```python
from build123d import *

# Parameters (mm, degrees)
SCHIZZO1_W                   = 100
SCHIZZO1_H                   = 50
ESTRUSIONE_ESTRUSIONE1_DEPTH = 2
RACCORDO1_R                  = 1
RACCORDO2_R                  = 1
SCHIZZO2_W                   = 15
SCHIZZO2_H                   = 9
TAGLIO_ESTRUSIONE1_DEPTH     = 10


with BuildPart() as part:
    # Schizzo1 → Estrusione-Estrusione1 (new body)
    with BuildSketch(Plane(origin=(0, 0, 0), x_dir=(1, 0, 0), z_dir=(0, 1, 0))):
        Rectangle(SCHIZZO1_W, SCHIZZO1_H)
    extrude(amount=ESTRUSIONE_ESTRUSIONE1_DEPTH)

    # Raccordo1
    raccordo1_edges = [part.edges().sort_by_distance(p)[0] for p in [
        (0, 0, -25),
        (0, 2, -25),
    ]]
    fillet(raccordo1_edges, radius=RACCORDO1_R - 0.0001)  # a hair under: the kernel refuses the full size

    # Raccordo2
    raccordo2_edges = [part.edges().sort_by_distance(p)[0] for p in [
        (50, 0.292863929, -24.707136071),
        (50, 1.707136071, -24.707136071),
        (50, 0, 0.49995),
        (50, 2, 0.49995),
    ]]
    fillet(raccordo2_edges, radius=RACCORDO2_R - 0.0001)  # a hair under: the kernel refuses the full size

    # Schizzo2 → Taglio-Estrusione1 (cut)
    with BuildSketch(Plane(origin=(0, 2, 0), x_dir=(1, 0, 0), z_dir=(0, 1, 0))):
        with Locations((-0.220921897, -5.005960214)):
            Rectangle(SCHIZZO2_W, SCHIZZO2_H)
    extrude(amount=-TAGLIO_ESTRUSIONE1_DEPTH, mode=Mode.SUBTRACT)


solid = part.part
```
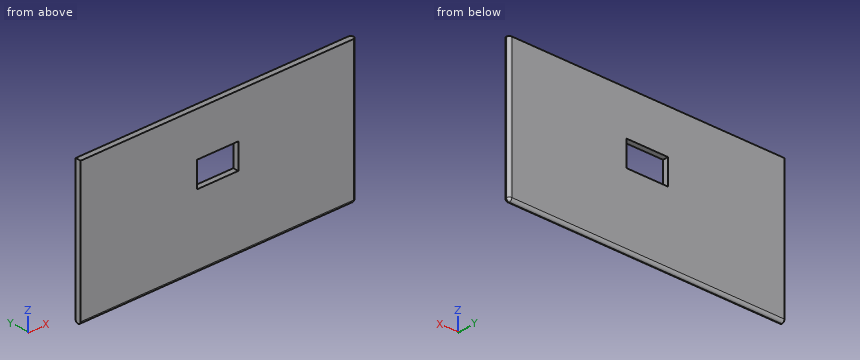
The listing builds one solid part. Answer for the finished solid, in the listing's coordinates (mm). Coordinates: 2 decimals unless noted, no trailing zeros. Write each loop counter-clockwise with the first axis right and the second up, starting at its lowest first coordinate (ties: lowest second). Pieces come first, ordered by that corner, then holes.
Q1. Find the intervals of material crossed by line 1 along X through (y, z) = (0.85, 7); line 2 along Z through (x, y) = (23, 0.85); line 3 along X through (y, z) = (0.25, 9), in increasing order.
Returned:
line 1: x = -50 to -7.72, 7.28 to 49.99
line 2: z = -24.99 to 25
line 3: x = -50 to -7.72, 7.28 to 49.66
Q2. Section B-B, the plane y = 1.6 is taken. Write down the section's boundary in (x, z).
Returned:
outline: (-50, -24.8) - (49, -24.8) arc R0.8 ccw to (49.8, -24) - (49.8, 25) - (-50, 25) - close; hole (-7.72, 0.51) - (7.28, 0.51) - (7.28, 9.51) - (-7.72, 9.51) - close
Q3. Given P1, Ø1, axis at x = -1, y = 0.5, coming from the -Z side, flat-ended and moving along its own axis, determine where the tip first touches the part or whether it passes through.
Returned:
P1: stops at z = -25
